Drawing for the job (mm, zero at the part's lowest x, y, z). Coordinates: 2 decimals unless noted, no trailing zeros. Order: outer loops, then holes, each group sorted by start corner. A loop starts at its lowest first (then second) coordinate and runs counter-clockwise, first axis right, second up.
1) Cut at A-A (x = 152.4). List the corners of the cut face in (y, z).
2) Pin check, flat tips, straight feed: pin 1 Ø10 at (x, z) = (151.5, 52) entering from +Y; pin 2 Ø3 at (x, y) = (222, 17) entering from +Z; pin 3 Ø5 at (y, z) = (15, 157) entering from +X. Stop position of each tip, or through.
3) Cut at C-C (y = 13.75). List the corners of the cut face in (x, z), and give its area (3 significant figures).
4) Cut at B-B (z = 203.2). List the corners of the cut face in (x, y).
5) Wall check: L1, parallel to X at y = 21.5, z = 50.8; L2, parallel to Z at x = 19.05, y = 20.75; L3, parallel to Z at x = 152.4, y = 23.25. Give the ranges that are in metal, low to high.
6) Cut at D-D (z = 164). List the corners of the cut face in (x, y).
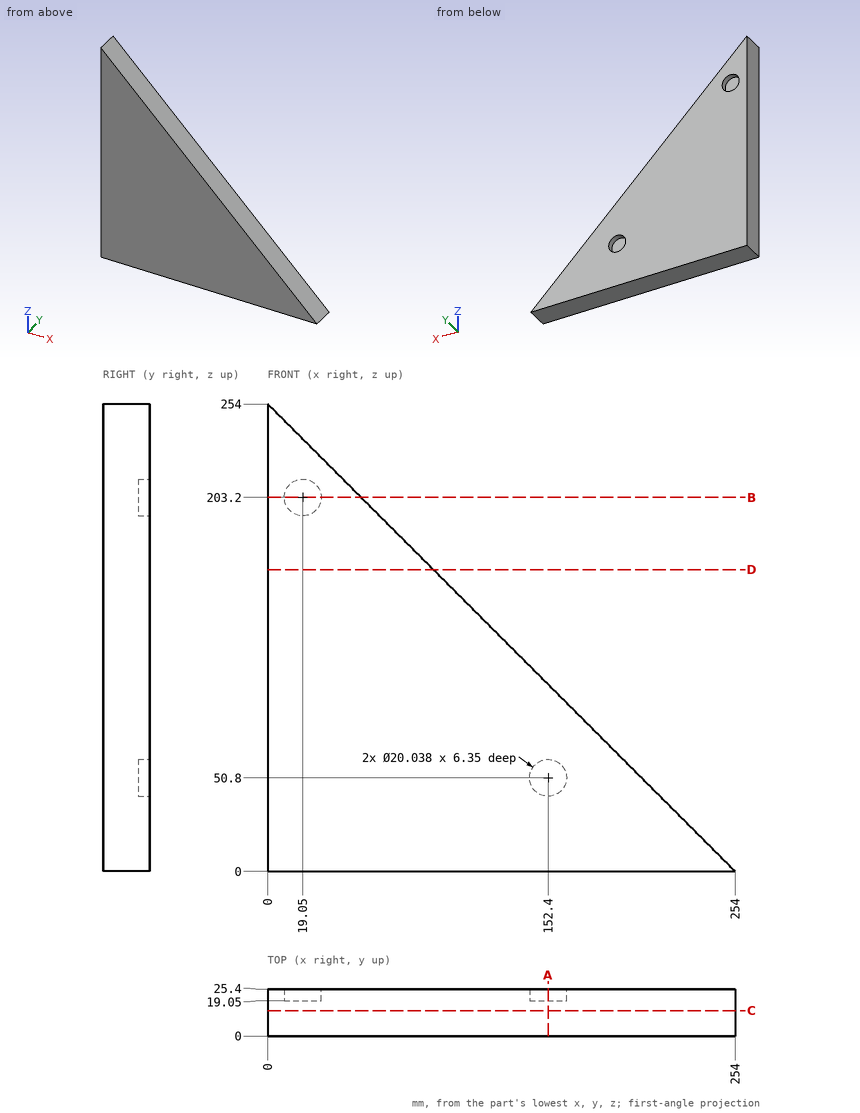
Geometry check:
1. outline: (0, 0) - (25.4, 0) - (25.4, 40.78) - (19.05, 40.78) - (19.05, 60.82) - (25.4, 60.82) - (25.4, 101.6) - (0, 101.6) - close
2. pin 1: stops at y = 19.05
2. pin 2: stops at z = 33.5
2. pin 3: stops at x = 99.5
3. outline: (0, 0) - (254, 0) - (0, 254) - close
3. area: 32,300 mm2
4. outline: (0, 0) - (50.8, 0) - (50.8, 25.4) - (29.07, 25.4) - (29.07, 19.05) - (9.03, 19.05) - (9.03, 25.4) - (0, 25.4) - close
5. L1: x = 0 to 142.38, 162.42 to 203.2
5. L2: z = 0 to 193.18, 213.22 to 234.95
5. L3: z = 0 to 40.78, 60.82 to 101.6
6. outline: (0, 0) - (90, 0) - (90, 25.4) - (0, 25.4) - close
